from build123d import *

# Parameters (mm, degrees)
F0_W     = 140
F0_H     = 30
F1_DEPTH = 15
F2_R     = 5
F3_W     = 47.9276580736
F3_H     = 20
F4_DEPTH = 25
F5_R     = 5
F6_R     = 5
F8_DEPTH = 25
F7_W     = 7.5194314122
F7_H     = 6.4587649889
F7_W_2   = 7.6362714171
F9_DEPTH = 5


with BuildPart() as f1:
    # F0 (on Top) → F1 (new body)
    with BuildSketch(Plane.XY):
        with Locations((11.6495971382, 1.335599795)):
            Rectangle(F0_W, F0_H)
    extrude(amount=F1_DEPTH)

    # F2
    f2_edges = [f1.edges().sort_by_distance(p)[0] for p in [
        (81.649597, -13.6644, 7.5),
        (81.649597, 16.3356, 7.5),
        (81.649597, 1.3356, 15),
        (11.649597, -13.6644, 15),
        (11.649597, 16.3356, 15),
    ]]
    fillet(f2_edges, radius=F2_R)

    # F3 (on face) → F4 (cut)
    with BuildSketch(Plane.XY.offset(15)):
        with Locations((11.0180326737, 1.335599795)):
            Rectangle(F3_W, F3_H)
    extrude(amount=-F4_DEPTH, mode=Mode.SUBTRACT)

    # F5
    f5_edges = [f1.edges().sort_by_distance(p)[0] for p in [
        (-12.945796, 1.3356, 15),
        (34.981862, 1.3356, 15),
    ]]
    fillet(f5_edges, radius=F5_R)

    # F6
    f6_edges = [f1.edges().sort_by_distance(p)[0] for p in [
        (-58.350403, 1.3356, 15),
    ]]
    fillet(f6_edges, radius=F6_R)

    # F7 (on face) → F8 (cut)
    with BuildSketch(Plane.XY.offset(15)):
        Polygon((73.7369505465, 1.335599795), (73.7369505465, 8.335599795), (49.7369505465, 8.335599795), (49.7369505465, 1.335599795), (49.7369505465, -5.664400205), (73.7369505465, -5.664400205), align=None)
    extrude(amount=-F8_DEPTH, mode=Mode.SUBTRACT)

    # F7 (on face) → F9 (cut)
    with BuildSketch(Plane.XY.offset(15)):
        Polygon((-53.3504028618, 1.335599795), (-53.3504028618, -2.2056352161), (-39.2847135663, -2.2056352161), (-31.6484421492, -2.2056352161), (-17.9457963631, -2.2056352161), (-17.9457963631, 1.335599795), (-17.9457963631, 4.8768348061), (-31.6484421492, 4.8768348061), (-39.1678735614, 4.8768348061), (-53.3504028618, 4.8768348061), align=None)
        with Locations((-35.4081578553, 8.1062173005)):
            Rectangle(F7_W, F7_H)
        with Locations((-35.4665778577, -5.4350177106)):
            Rectangle(F7_W_2, F7_H)
    extrude(amount=-F9_DEPTH, mode=Mode.SUBTRACT)


solid = f1.part
Could you check a few things on this model? Use its own coordinates, in mm. A direction names the side the tool comes from. Round coordinates to 2 decimals unless told otherwise and drop trailing zeros. Write each loop counter-clockwise with the first axis right and the second up, starting at its lowest first coordinate (ties: lowest second). Pieces come first, ordered by that corner, then holes. Notation, with made-up numbers: (87, 49.25) - (111, 49.25) arc R11 cw to (111, 54.25) - close; hole circle Ø11 at (-38, 58.5). An arc over 180 degrees is marked (long way). Put each result on its own line as item: value. Start each with the question number.
(1) I want a section at B-B, the plane z = 7.75. Please give me the cut outline in (x, y).
(2) I want a section at A-A, the plane x = 19.5. Please give me the cut outline in (y, z), plus the area to 3 significant figures.
(3) I want a section at D-D, the plane x = -41. Please give me the cut outline in (y, z).
(4) For faces 5 (the cylindrical face through (-14.449, 1.476, 13.574)), 6 (the flat face through (-12.946, 1, 5)), 7 (the cylindrical face through (-56.925, 14.832, 4.93)), which set-ups out of +Z, -Z, +X, -X, +Y, -Y let a thin tool reach every point of the face, with its end or its side?
(5) Will these pins go through, and if not, where does the flat tip stop? pin 1 (5.5 mm diameter, centred on y = 8.5, z = 12, fed in from +X); pin 2 (2.5 mm diameter, centred on x = -33.5, z = 12.5, fed in from +Y); pin 3 (2.5 mm diameter, centred on x = -22.5, z = 12.5, fed in from -Y); pin 4 (2.5 mm diameter, centred on x = -22.5, z = 12, fed in from +Y).
(6) I need wall thicknesses on probe 1 along X at (y, z) = (5.75, 4.5); probe 2 along Y at (x, z) = (-10.5, 6.75); probe 3 along Y at (x, z) = (61, 2). Which ranges of each line are inside material? Lowest first, please.
(7) I want a section at C-C, the plane x = 64.5. Please give me the cut outline in (y, z), plus the area to 3 significant figures.
(8) Thinking about a two-plate mould opening in Y: for faces 1 (the cylindrical face through (36.485, 1.476, 13.574)), 2 (the flat face through (11, -13.664, 5)), 3 (the flat face through (49.737, 1, 8)), 4 (the cylindrical face through (-56.92, 1.48, 13.5)), which applies, released by +Y, released by -Y, zero draft, split by the parting line, or undercut?
Here are the results:
1. outline: (-58.35, -8.66) arc R5 ccw to (-53.35, -13.66) - (76.65, -13.66) arc R5 ccw to (81.65, -8.66) - (81.65, 11.34) arc R5 ccw to (76.65, 16.34) - (-53.35, 16.34) arc R5 ccw to (-58.35, 11.34) - close; hole (-12.95, -8.66) - (34.98, -8.66) - (34.98, 11.34) - (-12.95, 11.34) - close; hole (49.74, -5.66) - (73.74, -5.66) - (73.74, 8.34) - (49.74, 8.34) - close
2. outline: (-13.66, 0) - (-8.66, 0) - (-8.66, 15) arc R5 ccw to (-13.66, 10) - close; (11.34, 0) - (16.34, 0) - (16.34, 10) arc R5 ccw to (11.34, 15) - close
2. area: 139 mm^2
3. outline: (-13.66, 0) - (16.34, 0) - (16.34, 10) arc R5 ccw to (11.34, 15) - (4.88, 15) - (4.88, 10) - (-2.21, 10) - (-2.21, 15) - (-8.66, 15) arc R5 ccw to (-13.66, 10) - close
4. face 5: +Z
4. face 6: +Z, -Z
4. face 7: +Z, -Z, -X, +Y
5. pin 1: stops at x = 81.65
5. pin 2: stops at y = 16.18
5. pin 3: stops at y = -13.51
5. pin 4: stops at y = 16.28
6. probe 1: x = -58.35 to -12.95, 34.98 to 49.74, 73.74 to 81.65
6. probe 2: y = -13.66 to -8.66, 11.34 to 16.34
6. probe 3: y = -13.66 to -5.66, 8.34 to 16.34
7. outline: (-13.66, 0) - (-5.66, 0) - (-5.66, 15) - (-8.66, 15) arc R5 ccw to (-13.66, 10) - close; (8.34, 0) - (16.34, 0) - (16.34, 10) arc R5 ccw to (11.34, 15) - (8.34, 15) - close
7. area: 229 mm^2
8. face 1: undercut
8. face 2: released by -Y
8. face 3: undercut
8. face 4: zero draft
